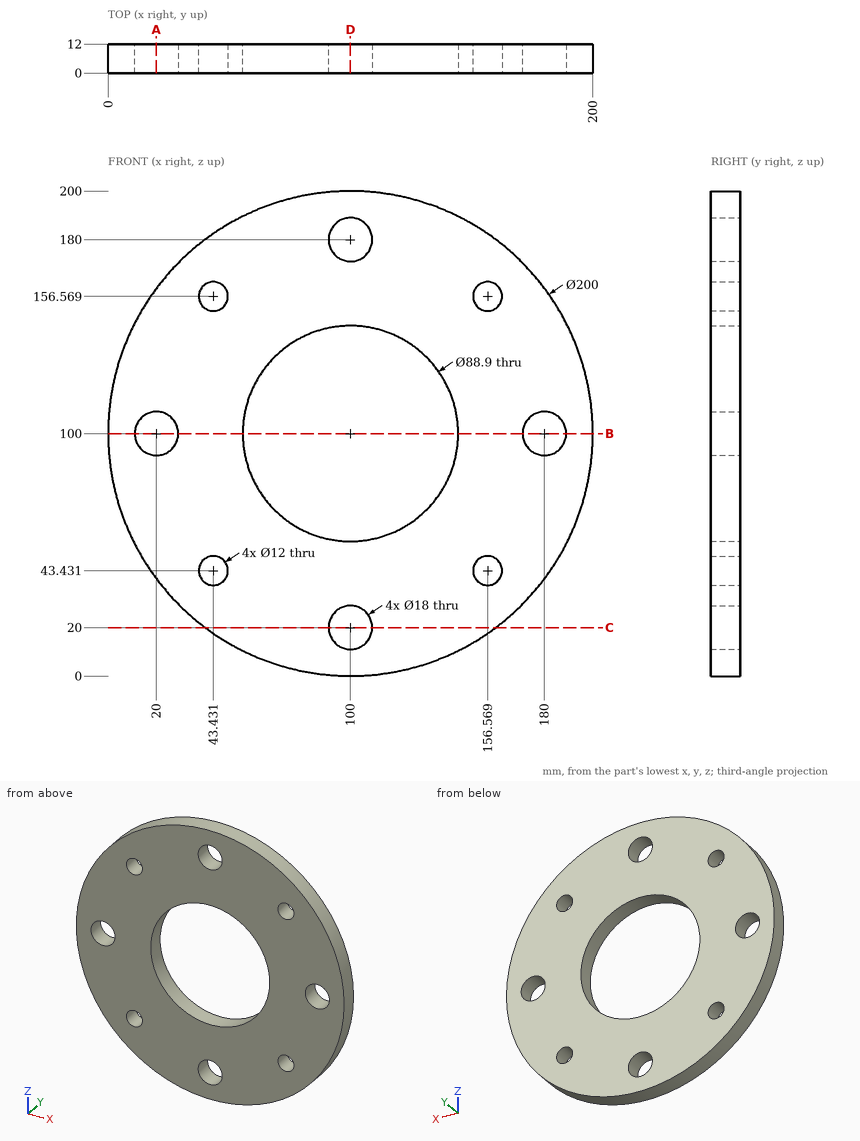
Design review of the part shown in the three views and the two pictorial views. Dimensions are in mm from the part's minimum x, y and z. Round coordinates to 2 decimals unless told otherwise and drop trailing zeros. Order: outer loops, then holes, each group sorted by start corner. A loop starts at its lowest first (then second) coordinate and runs counter-clockwise, first axis right, second up.
Item 1: To check wall thickness, follow probe 1 along Z at (x, y) = (100.5, 5); probe 2 along Z at (x, y) = (47, 2) (1 decimal); probe 3 along Z at (x, y) = (161, 3.5) (1 decimal). State the ranges of each line that lie inside material, in increasing order.
Working result:
probe 1: z = 0 to 11.01, 28.99 to 55.55, 144.45 to 171.01, 188.99 to 200
probe 2: z = 15.2 to 38.6, 48.3 to 151.7, 161.4 to 184.8
probe 3: z = 20.8 to 39.4, 47.5 to 152.5, 160.6 to 179.2
Item 2: Add section A-A, the plane x = 20. State the section outline as (y, z) points, and give its area (3 significant figures).
Working result:
outline: (0, 40) - (12, 40) - (12, 91) - (0, 91) - close; (0, 109) - (12, 109) - (12, 160) - (0, 160) - close
area: 1,220 mm2
Item 3: Add section B-B, the plane z = 100. State the section outline as (x, y) points.
Working result:
outline: (0, 0) - (11, 0) - (11, 12) - (0, 12) - close; (29, 0) - (55.55, 0) - (55.55, 12) - (29, 12) - close; (144.45, 0) - (171, 0) - (171, 12) - (144.45, 12) - close; (189, 0) - (200, 0) - (200, 12) - (189, 12) - close
Item 4: Add section C-C, the plane z = 20. State the section outline as (x, y) points, and give its area (3 significant figures).
Working result:
outline: (40, 0) - (91, 0) - (91, 12) - (40, 12) - close; (109, 0) - (160, 0) - (160, 12) - (109, 12) - close
area: 1,220 mm2
Item 5: Add section D-D, the plane x = 100. State the section outline as (y, z) points.
Working result:
outline: (0, 0) - (12, 0) - (12, 11) - (0, 11) - close; (0, 29) - (12, 29) - (12, 55.55) - (0, 55.55) - close; (0, 144.45) - (12, 144.45) - (12, 171) - (0, 171) - close; (0, 189) - (12, 189) - (12, 200) - (0, 200) - close
Item 6: For pin 1 (3 mm diameter, centred on x = 168.5, y = 4.5, fed in from -Z) (1 decimal); pin 2 (1.5 mm diameter, centred on y = 3.5, z = 58, fed in from -X) (1 decimal), all flat-tipped, find the tip position at first contact; note any pin that passes through.
Working result:
pin 1: stops at z = 25.8
pin 2: stops at x = 8.9
